```python
from build123d import *

# Parameters (mm, degrees)
CYLINDER031_R               = 5
CYLINDER031_DEPTH           = 3
CYLINDER028_R               = 9.25
CYLINDER028_DEPTH           = 3
CYLINDER029_R               = 6
CYLINDER029_DEPTH           = 9
CYLINDER030_R               = 9.25
CYLINDER030_DEPTH           = 9
CYLINDER030_PLACEMENT_ANGLE = 1


with BuildPart() as smallplughole:
    # Cylinder031 → Cylinder031 (new body)
    with BuildSketch(Plane.XY):
        Circle(CYLINDER031_R)
    extrude(amount=CYLINDER031_DEPTH)


with BuildPart() as smallplugbas:
    # Cylinder028 → Cylinder028 (new body)
    with BuildSketch(Plane.XY):
        Circle(CYLINDER028_R)
    extrude(amount=CYLINDER028_DEPTH)

    # Cut011: cut SmallPlugHole
    add(smallplughole.part, mode=Mode.SUBTRACT)


with BuildPart() as smallplugwallhole:
    # Cylinder029 → Cylinder029 (new body)
    with BuildSketch(Plane.XY.offset(2.5)):
        Circle(CYLINDER029_R)
    extrude(amount=CYLINDER029_DEPTH)


with BuildPart() as obj1:
    # Cylinder030 → Cylinder030 (new body)
    with BuildSketch(Plane.XY):
        Circle(CYLINDER030_R)
    extrude(amount=CYLINDER030_DEPTH)


with BuildPart() as obj1_1:
    # Cylinder030 placement: moved
    add(obj1.part.moved(Location((0, 0, 2.5))).rotate(Axis((0, 0, 2.5), (0, 0, 1)), CYLINDER030_PLACEMENT_ANGLE))

    # Cut010: cut SmallPlugWallHole
    add(smallplugwallhole.part, mode=Mode.SUBTRACT)

    # Fusion023: union SmallPlugBas
    add(smallplugbas.part)


with BuildPart() as obj1_2:
    # Fusion023 placement: moved
    add(obj1_1.part.moved(Location((54, -192.254, 94))))


solid = obj1_2.part
```
The listing builds one solid part. Answer for the finished solid, in the listing's coordinates (mm). A direction names the side the tool comes from. Round coordinates to 2 decimals unless told otherwise and drop trailing zeros. Loops run counter-clockwise (first coordinate to the right, second up) from the corner with the lowest first, then second, coordinate; pieces in that order, holes last.
Q1. Given pin 1 Ø6 at (x, z) = (58, 100) entering from +Y; pin 2 Ø2 at (x, z) = (56.5, 104) entering from -Y; pin 3 Ø2 at (x, z) = (52.5, 95.5) entering from -Y, each flat-ended and moving along its own axis, determine where each tip first touches the part or whether it passes through.
Q2. Section C-C, the plane z = 100.25 is taken. Determine the outline of the cut face in (x, y), then the cut area to 3 significant figures.
Q3. Section A-A, the plane x = 54 is taken. Determine the outline of the cut face in (y, z), then the cut area to 4 significant figures.
Q4. Section B-B, the plane y = -193 is taken. Determine the outline of the cut face in (x, z).
Q5. Find the intervals of material crossed by line 1 (Y direction, x = 54, z = 95); line 2 (Y direction, x = 54, z = 100); line 3 (Z direction, x = 48.5, y = -193.5), in increasing order.
Q6. Which of the six approach directions +Z, -Z, +X, -X, +Y, -Y give full straight-line access (tool end or side, diameter ignored) to faces 5 (the face through (53, -187, 97)), 6 (the face through (58, -196, 94))?
Q7. For a pull along X with two mould halves and no side action, classify faces 1 (the face through (56, -198.3, 105.5)), 2 (the face through (62.82, -189.47, 99.67)), 3 (the face through (53.349, -187.297, 95.479)), 4 (the face through (49.578, -188.199, 101.19)) as released by +X, released by -X, zero draft, split by the parting line, or undercut.
Q8. Section D-D, the plane y = -185.75 is taken. Determine the outline of the cut face in (x, z), then the cut area to 3 significant figures.
Completed:
1. pin 1: stops at y = -183.06
1. pin 2: stops at y = -201.38
1. pin 3: stops at y = -201.49
2. outline: circle Ø18.5 at (54, -192.25); hole circle Ø12 at (54, -192.25)
2. area: 156 mm2
3. outline: (-201.5, 94) - (-197.25, 94) - (-197.25, 97) - (-198.25, 97) - (-198.25, 105.5) - (-201.5, 105.5) - close; (-187.25, 94) - (-183, 94) - (-183, 105.5) - (-186.25, 105.5) - (-186.25, 97) - (-187.25, 97) - close
3. area: 80.75 mm2
4. outline: (44.78, 94) - (49.06, 94) - (49.06, 97) - (48.05, 97) - (48.05, 105.5) - (44.78, 105.5) - close; (58.94, 94) - (63.22, 94) - (63.22, 105.5) - (59.95, 105.5) - (59.95, 97) - (58.94, 97) - close
5. line 1: y = -201.5 to -197.25, -187.25 to -183
5. line 2: y = -201.5 to -198.25, -186.25 to -183
5. line 3: z = 94 to 97
6. face 5: +Z
6. face 6: -Z, +X, -X, +Y, -Y
7. face 1: zero draft
7. face 2: split by the parting line
7. face 3: undercut
7. face 4: undercut
8. outline: (47.42, 94) - (60.58, 94) - (60.58, 105.5) - (47.42, 105.5) - close
8. area: 151 mm2
